For this review, take the finished solid that the model builds, in its own axes (mm). A direction names the side the tool comes from. Round coordinates to 2 decimals unless told otherwise and drop trailing zeros. Order: outer loops, then holes, each group sorted by start corner. A loop starts at its lowest first (then second) coordinate and runs counter-clockwise, first axis right, second up.
```python
from build123d import *

# Parameters (mm, degrees)
SKETCH1_R                    = 1.8288
BASE_FLANGE1_DEPTH           = 1.016
EDGE_FLANGE1_STRIP_W         = 5.6515
EDGE_FLANGE1_STRIP_H         = 1.016
EDGE_FLANGE1_STRIP_CUT_DEPTH = 11.1125
EDGE_FLANGE1_DEPTH           = 11.1125
FILLET1_R                    = 4.7625


# Sheet-metal steps are written as plain solids
with BuildPart() as part:
    # Sketch1 → Base-Flange1 (new body)
    with BuildSketch(Plane.XY):
        with BuildLine():
            Line((-12.7, 65.88125), (-6.35, 65.88125))
            Line((-6.35, 65.88125), (-6.35, 54.76875))
            Line((-6.35, 54.76875), (-12.7, 54.76875))
            ThreePointArc((-12.7, 54.76875), (-18.25625, 60.325), (-12.7, 65.88125))
        make_face()
        with Locations((-12.7, 60.325)):
            Circle(SKETCH1_R, mode=Mode.SUBTRACT)
    extrude(amount=BASE_FLANGE1_DEPTH)

    # Edge-Flange1 strip (across the edge) → Edge-Flange1 strip cut (cut)
    with BuildSketch(Plane(origin=(-6.35, 54.76875, 1.016), x_dir=(-1, 0, 0), z_dir=(0, 1, 0))):
        with Locations((-1.016, -0.508)):
            Rectangle(EDGE_FLANGE1_STRIP_W, EDGE_FLANGE1_STRIP_H)
    extrude(amount=EDGE_FLANGE1_STRIP_CUT_DEPTH, mode=Mode.SUBTRACT)

    # Edge-Flange1 section (across the edge) → Edge-Flange1 (add)
    with BuildSketch(Plane(origin=(-6.35, 54.76875, 1.016), x_dir=(-1, 0, 0), z_dir=(0, 1, 0))):
        with BuildLine():
            Line((0, 0.79375), (0, 20.32))
            Line((0, 20.32), (1.016, 20.32))
            Line((1.016, 20.32), (1.016, 0.79375))
            ThreePointArc((1.016, 0.79375), (1.248483992, 0.232483992), (1.80975, 0))
            Line((1.80975, 0), (1.80975, -1.016))
            ThreePointArc((1.80975, -1.016), (0.530063503, -0.485936497), (0, 0.79375))
        make_face()
    extrude(amount=EDGE_FLANGE1_DEPTH)

    # Fillet1
    fillet1_edges = [part.edges().sort_by_distance(p)[0] for p in [
        (-6.858, 54.76875, 21.336),
        (-6.858, 65.88125, 21.336),
    ]]
    fillet(fillet1_edges, radius=FILLET1_R)


solid = part.part
```
Q1. Take a section at B-B, the plane z = 15.25. State the section outline as (x, y) points.
Q2. Mouldability with a two-part tool opening along Y and no side actions: class faces 3 (the face through (-11.86, 58.7, 0.5)), 4 (the face through (-6.35, 60, 11)), 5 (the face through (-18.255, 60.203, 0.501)), 6 (the face through (-7, 54.769, 6)) as +Y half, -Y half, draft (parallel to the pull), parting line (faces both ways), or undercut.
Q3. Take a section at D-D, the plane x = -8.5. State the section outline as (y, z) points.
Q4. Take a section at A-A, the plane x = -11.75. State the section outline as (y, z) points, plus the area to 3 significant figures.
Q5. Wall thickness on line 1 (Y direction, x = -12.7, z = 0.6); line 2 (X direction, y = 63.5, z = 18.25); line 3 (Z direction, x = -9.25, y = 62.25): over which ranges is each line inside the solid? List them lowest first.
Q6. Take a section at C-C, the plane y = 63.25. State the section outline as (x, z) points, plus the area to 3 significant figures.
Q7. Tool access review of faces 1 (the face through (-7.366, 60, 12)), 2 (the face through (-6.865, 64.449, 19.978)): name each direction out of +Z, -Z, +X, -X, +Y, -Y from which nothing blocks a thin tool from reaching the whole face with its end or side.
Q8. Clearance check with flat-ended pins moving along their axes: pin 1 (5 mm diameter, centred on x = -14, y = 58.5, fed in from +Z); pin 2 (1.5 mm diameter, centred on y = 62, z = 15, fed in from -X); pin 3 (1 mm diameter, centred on x = -9.5, z = 15.5, fed in from -Y). State where each tip first meets the part, or that it passes through.
Working result:
1. outline: (-7.37, 54.77) - (-6.35, 54.77) - (-6.35, 65.88) - (-7.37, 65.88) - close
2. face 3: undercut
2. face 4: draft
2. face 5: parting line
2. face 6: -Y half
3. outline: (54.77, 0) - (65.88, 0) - (65.88, 1.02) - (54.77, 1.02) - close
4. outline: (54.77, 0) - (58.76, 0) - (58.76, 1.02) - (54.77, 1.02) - close; (61.89, 0) - (65.88, 0) - (65.88, 1.02) - (61.89, 1.02) - close
4. area: 8.11 mm2
5. line 1: y = 54.77 to 58.5, 62.15 to 65.88
5. line 2: x = -7.37 to -6.35
5. line 3: z = 0 to 1.02
6. outline: (-17.42, 0) - (-8.16, 0) arc R1.81 ccw to (-6.35, 1.81) - (-6.35, 20.83) - (-7.37, 20.83) - (-7.37, 1.81) arc R0.79 cw to (-8.16, 1.02) - (-17.42, 1.02) - close
6. area: 30.8 mm2
7. face 1: +Z, -X, +Y, -Y
7. face 2: +Z, +X, -X, +Y
8. pin 1: stops at z = 1.02
8. pin 2: stops at x = -7.37
8. pin 3: passes through
